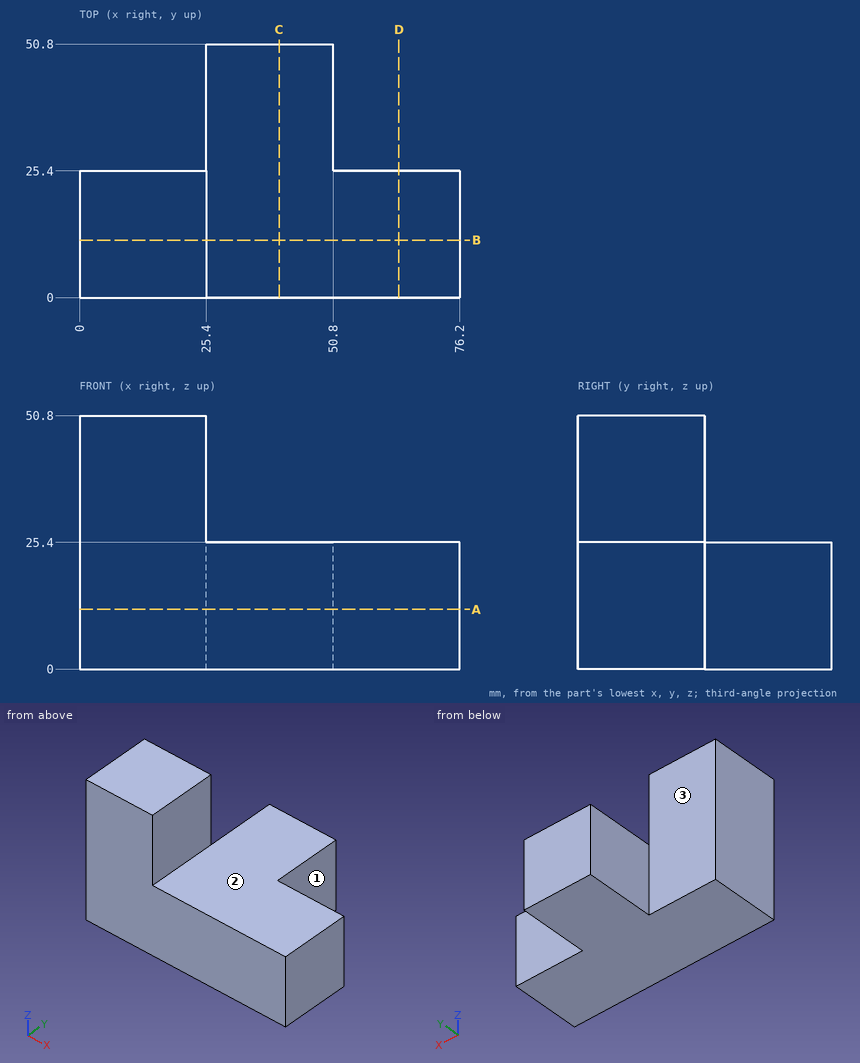
Verification items for this drawing (mm, ordinates from the low corner). A direction names the side the tool comes from. Round coordinates to 2 decimals unless told otherwise and drop trailing zeros. Order: outer loops, then holes, each group sorted by start corner. A loop starts at its lowest first (then second) coordinate and runs counter-clockwise, first axis right, second up. Notation, with made-up numbers: (76.25, 6) - (85.25, 6) arc R30 cw to (85.25, 45) - close; hole circle Ø7 at (48.25, 57). An arc over 180 degrees is marked (long way). Answer as CSV lines item,"result". Start each with the question number.
1) Depth check by flat-ended pin: pin 1 (12 mm diameter, centred on y = 30.5, z = 15.5, fed in from +X); pin 2 (7.5 mm diameter, centred on x = 10, z = 16.5, fed in from +Y); pin 3 (15 mm diameter, centred on x = 52, y = 32.5, fed in from +Z); pin 4 (10 mm diameter, centred on y = 45, z = 13.5, fed in from +X). Enter the tip coordinate at first touch or a pass-through.
2) Scan lines: probe 1 along X at (y, z) = (45.5, 17); probe 2 along Y at (x, z) = (9, 40). Record each from-to range of solid material in increasing order.
3) Section check A-A (z = 12). Record the cut outline in (x, y).
4) Section check D-D (x = 64). Record the cut outline in (y, z), then the cut area to 3 significant figures.
5) Section check B-B (y = 11.5). Record the cut outline in (x, z).
6) Tool access check on the marked faces 1, 2 and 3. Record the directions out of +Z, -Z, +X, -X, +Y, -Y that give a thin tool (end or side, any length) a straight path to the whole face; none if there is none.
7) Section check C-C (x = 40). Record the cut outline in (y, z).
Determined:
1,pin 1,"x = 76.2"
1,pin 2,"y = 25.4"
1,pin 3,"z = 25.4"
1,pin 4,"x = 50.8"
2,probe 1,"25.4 to 50.8"
2,probe 2,"0 to 25.4"
3,outline,"(0, 0) - (76.2, 0) - (76.2, 25.4) - (50.8, 25.4) - (50.8, 50.8) - (25.4, 50.8) - (25.4, 25.4) - (0, 25.4) - close"
4,outline,"(0, 0) - (25.4, 0) - (25.4, 25.4) - (0, 25.4) - close"
4,area,"645 mm^2"
5,outline,"(0, 0) - (76.2, 0) - (76.2, 25.4) - (25.4, 25.4) - (25.4, 50.8) - (0, 50.8) - close"
6,face 1,"+Z, -Z, +X, +Y"
6,face 2,"+Z, +X, +Y, -Y"
6,face 3,"+Z, -Z, -X, +Y"
7,outline,"(0, 0) - (50.8, 0) - (50.8, 25.4) - (0, 25.4) - close"
